```python
from build123d import *

# Parameters (mm, degrees)
F0_R     = 1.5
F0_R_2   = 11
F0_R_3   = 4.65
F0_R_4   = 2.5
F1_DEPTH = 48
F2_START = -8
F2_DEPTH = 31
F3_DEPTH = 2
F4_DEPTH = 12
F5_DEPTH = 4.5


with BuildPart() as f1:
    # F0 (on Top) → F1 (new body)
    with BuildSketch(Plane.XY):
        with BuildLine():
            Line((-13.5532984915, -21.15), (13.5532984915, -21.15))
            ThreePointArc((13.5532984915, -21.15), (17.7625223434, -17.7625223434), (21.15, -13.5532984915))
            Line((21.15, -13.5532984915), (21.15, 13.5532984915))
            ThreePointArc((21.15, 13.5532984915), (17.7625223434, 17.7625223434), (13.5532984915, 21.15))
            Line((13.5532984915, 21.15), (-13.5532984915, 21.15))
            ThreePointArc((-13.5532984915, 21.15), (-17.7625223434, 17.7625223434), (-21.15, 13.5532984915))
            Line((-21.15, 13.5532984915), (-21.15, -13.5532984915))
            ThreePointArc((-21.15, -13.5532984915), (-17.7625223434, -17.7625223434), (-13.5532984915, -21.15))
        make_face()
        with Locations((-15.5, -15.5)):
            Circle(F0_R, mode=Mode.SUBTRACT)
        with Locations((15.5, -15.5)):
            Circle(F0_R, mode=Mode.SUBTRACT)
        with Locations((-15.5, 15.5)):
            Circle(F0_R, mode=Mode.SUBTRACT)
        Circle(F0_R_2, mode=Mode.SUBTRACT)
        with Locations((15.5, 15.5)):
            Circle(F0_R, mode=Mode.SUBTRACT)
        Circle(F0_R_2)
        Circle(F0_R_3, mode=Mode.SUBTRACT)
        with Locations((-15.5, 15.5)):
            Circle(F0_R)
        with Locations((15.5, 15.5)):
            Circle(F0_R)
        with Locations((15.5, -15.5)):
            Circle(F0_R)
        with Locations((-15.5, -15.5)):
            Circle(F0_R)
        Circle(F0_R_3)
        Circle(F0_R_4, mode=Mode.SUBTRACT)
        Circle(F0_R_4)
        with BuildLine():
            ThreePointArc((13.5532984915, 21.15), (17.7625223434, 17.7625223434), (21.15, 13.5532984915))
            Line((21.15, 13.5532984915), (21.15, 16.6865544676))
            ThreePointArc((21.15, 16.6865544676), (19.0494566852, 19.0494566852), (16.6865544676, 21.15))
            Line((16.6865544676, 21.15), (13.5532984915, 21.15))
        make_face()
        with BuildLine():
            ThreePointArc((-16.6865544676, 21.15), (-19.0494566852, 19.0494566852), (-21.15, 16.6865544676))
            Line((-21.15, 16.6865544676), (-21.15, 13.5532984915))
            ThreePointArc((-21.15, 13.5532984915), (-17.7625223434, 17.7625223434), (-13.5532984915, 21.15))
            Line((-13.5532984915, 21.15), (-16.6865544676, 21.15))
        make_face()
        with BuildLine():
            ThreePointArc((-21.15, -16.6865544676), (-19.0494566852, -19.0494566852), (-16.6865544676, -21.15))
            Line((-16.6865544676, -21.15), (-13.5532984915, -21.15))
            ThreePointArc((-13.5532984915, -21.15), (-17.7625223434, -17.7625223434), (-21.15, -13.5532984915))
            Line((-21.15, -13.5532984915), (-21.15, -16.6865544676))
        make_face()
        with BuildLine():
            Line((13.5532984915, -21.15), (16.6865544676, -21.15))
            ThreePointArc((16.6865544676, -21.15), (19.0494566852, -19.0494566852), (21.15, -16.6865544676))
            Line((21.15, -16.6865544676), (21.15, -13.5532984915))
            ThreePointArc((21.15, -13.5532984915), (17.7625223434, -17.7625223434), (13.5532984915, -21.15))
        make_face()
    extrude(amount=-F1_DEPTH)

    # F0 (on Top) → F2 (cut)
    with BuildSketch(Plane.XY.offset(F2_START)):
        with BuildLine():
            ThreePointArc((-16.6865544676, 21.15), (-19.0494566852, 19.0494566852), (-21.15, 16.6865544676))
            Line((-21.15, 16.6865544676), (-21.15, 13.5532984915))
            ThreePointArc((-21.15, 13.5532984915), (-17.7625223434, 17.7625223434), (-13.5532984915, 21.15))
            Line((-13.5532984915, 21.15), (-16.6865544676, 21.15))
        make_face()
        with BuildLine():
            ThreePointArc((-21.15, -16.6865544676), (-19.0494566852, -19.0494566852), (-16.6865544676, -21.15))
            Line((-16.6865544676, -21.15), (-13.5532984915, -21.15))
            ThreePointArc((-13.5532984915, -21.15), (-17.7625223434, -17.7625223434), (-21.15, -13.5532984915))
            Line((-21.15, -13.5532984915), (-21.15, -16.6865544676))
        make_face()
        with BuildLine():
            ThreePointArc((13.5532984915, 21.15), (17.7625223434, 17.7625223434), (21.15, 13.5532984915))
            Line((21.15, 13.5532984915), (21.15, 16.6865544676))
            ThreePointArc((21.15, 16.6865544676), (19.0494566852, 19.0494566852), (16.6865544676, 21.15))
            Line((16.6865544676, 21.15), (13.5532984915, 21.15))
        make_face()
        with BuildLine():
            Line((13.5532984915, -21.15), (16.6865544676, -21.15))
            ThreePointArc((16.6865544676, -21.15), (19.0494566852, -19.0494566852), (21.15, -16.6865544676))
            Line((21.15, -16.6865544676), (21.15, -13.5532984915))
            ThreePointArc((21.15, -13.5532984915), (17.7625223434, -17.7625223434), (13.5532984915, -21.15))
        make_face()
    extrude(amount=-F2_DEPTH, mode=Mode.SUBTRACT)

    # F0 (on Top) → F3 (join)
    with BuildSketch(Plane.XY):
        Circle(F0_R_2)
        Circle(F0_R_3, mode=Mode.SUBTRACT)
    extrude(amount=F3_DEPTH)

    # F0 (on Top) → F4 (join)
    with BuildSketch(Plane.XY):
        Circle(F0_R_4)
    extrude(amount=F4_DEPTH)

    # F0 (on Top) → F5 (cut)
    with BuildSketch(Plane.XY):
        with Locations((-15.5, 15.5)):
            Circle(F0_R)
        with Locations((15.5, 15.5)):
            Circle(F0_R)
        with Locations((15.5, -15.5)):
            Circle(F0_R)
        with Locations((-15.5, -15.5)):
            Circle(F0_R)
    extrude(amount=-F5_DEPTH, mode=Mode.SUBTRACT)


solid = f1.part
```
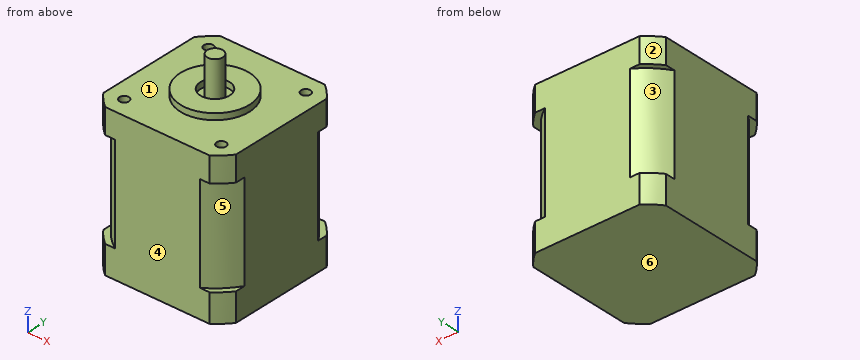
The listing builds one solid part. Answer for the finished solid, in the listing's coordinates (mm). Face numbers are marked on the shaded views. A direction names the side the tool comes from. Round coordinates to 2 decimals unless told otherwise and drop trailing zeros. Loops run counter-clockwise (first coordinate to the right, second up) from the corner with the lowest first, then second, coordinate; pieces in that order, holes last.
1) Given P1, Ø1.5, axis at x = -15, y = -1.5, coming from the +Z side; P2, Ø2.5, axis at x = -15.5, y = -15.5, coming from the +Z side; P3, Ø12, axis at x = -6, y = -8, coming from the +Z side, each flat-ended and moving along its own axis, determine where each tip first touches the part or whether it passes through.
Outcome:
P1: stops at z = 0
P2: stops at z = -4.5
P3: stops at z = 2
2) A cutting plane is placed at C-C on x = -0.5. Determine the outline of the cut face in (y, z), plus the area to 3 significant figures.
Outcome:
outline: (-21.15, -48) - (21.15, -48) - (21.15, 0) - (10.99, 0) - (10.99, 2) - (4.62, 2) - (4.62, 0) - (2.45, 0) - (2.45, 12) - (-2.45, 12) - (-2.45, 0) - (-4.62, 0) - (-4.62, 2) - (-10.99, 2) - (-10.99, 0) - (-21.15, 0) - close
area: 2,110 mm2
3) A cutting plane is placed at D-D on y = 15.5. Determine the outline of the cut face in (x, z), plus the area to 3 significant figures.
Outcome:
outline: (-21.15, -48) - (21.15, -48) - (21.15, -39) - (19.77, -39) - (19.77, -8) - (21.15, -8) - (21.15, 0) - (17, 0) - (17, -4.5) - (14, -4.5) - (14, 0) - (-14, 0) - (-14, -4.5) - (-17, -4.5) - (-17, 0) - (-21.15, 0) - (-21.15, -8) - (-19.77, -8) - (-19.77, -39) - (-21.15, -39) - close
area: 1,920 mm2
4) A cutting plane is placed at A-A on z = -2.5. Determine the outline of the cut face in (x, y), plus the area to 3 significant figures.
Outcome:
outline: (-21.15, -16.69) arc R26.94 ccw to (-16.69, -21.15) - (16.69, -21.15) arc R26.94 ccw to (21.15, -16.69) - (21.15, 16.69) arc R26.94 ccw to (16.69, 21.15) - (-16.69, 21.15) arc R26.94 ccw to (-21.15, 16.69) - close; hole circle Ø3 at (-15.5, -15.5); hole circle Ø3 at (-15.5, 15.5); hole circle Ø3 at (15.5, -15.5); hole circle Ø3 at (15.5, 15.5)
area: 1,720 mm2
5) For a pull along Z with two mould halves and no side action, classify the marked faces 4, 5 and 6 as released by +Z, released by -Z, zero draft, split by the parting line, or undercut.
Outcome:
face 4: zero draft
face 5: undercut
face 6: released by -Z
6) A cutting plane is placed at B-B on z = -41.5. Determine the outline of the cut face in (x, y), plus the area to 3 significant figures.
Outcome:
outline: (-21.15, -16.69) arc R26.94 ccw to (-16.69, -21.15) - (16.69, -21.15) arc R26.94 ccw to (21.15, -16.69) - (21.15, 16.69) arc R26.94 ccw to (16.69, 21.15) - (-16.69, 21.15) arc R26.94 ccw to (-21.15, 16.69) - close
area: 1,750 mm2
7) Consider line 1 (Y direction, x = 0, z = 0.4); line 2 (Y direction, x = -15, z = -1); line 3 (Z direction, x = -1, y = 15). Determine where each line is inside the solid, lowest interval first.
Outcome:
line 1: y = -11 to -4.65, -2.5 to 2.5, 4.65 to 11
line 2: y = -21.15 to -16.91, -14.09 to 14.09, 16.91 to 21.15
line 3: z = -48 to 0
8) For the marked faces 1, 2 and 3, determine the directions among +Z, -Z, +X, -X, +Y, -Y from which every point of the face is accessible in a straight line to the end or side of a thin tool.
Outcome:
face 1: +Z
face 2: +Z, -Z, -X, +Y
face 3: -X, +Y
